Source: CAD feature listing. Evaluate the final solid. Frame: model axes, mm. A direction names the side the tool comes from. Give positions to 0.01 mm unless a question says otherwise; leave off trailing zeros. Write each loop counter-clockwise with the first axis right and the second up, starting at its lowest first coordinate (ties: lowest second). Pieces come first, ordered by that corner, then holes. Notation, with made-up numbers: (53.25, 10.5) -> (84.25, 10.5) arc R28 cw to (84.25, 28.5) -> close; hole circle Ø4 at (63.5, 8.25). An arc over 180 degrees is marked (long way). Answer as a JSON object with one key per item and string values. Group by question number.
Item 1: Section query A-A on y = -3.75. Return the cut outline in (x, z).
Item 2: Ray query, probe 1 along Z at (x, y) = (-10.5, -0.85); probe 2 along X at (y, z) = (-1.85, 207); probe 3 along X at (y, z) = (-2.65, 72). Return the intervals inside material, ascending. Write a range as from..to.
Item 3: First-contact query: pin 1 Ø1.8 at (x, y) = (-14, -1.5) entering from -Z; pin 2 Ø1 at (y, z) = (-3, 9) entering from +X. Flat tips, straight axial feed; report the tip coordinate or a pass-through.
Item 4: Pull-direction query (Z, two-part tool) for faces 4 (the face through (-44, -3, 8)), 5 (the face through (-11, -3, 235)), 6 (the face through (-41, 0, 120)); classes: pulls with the +Z half, pulls with the -Z half, needs draft (parallel to the pull), parting line crosses it, or undercut.
Item 5: Section query B-B on x = -44.5. Return the cut outline in (y, z).
Item 6: Access query for faces 1 (the face through (-39.725, -2.958, 121.903)), 2 (the face through (-41, -3, 4)), 3 (the face through (-46.88, -2.96, 128.19)). Directions: +Z, -Z, +X, -X, +Y, -Y. A direction counts if a zero-diameter tool reaches every point of the face in a straight line with its end or side. Return the directions, or none.
Item 7: Section query C-C on x = -33. Return the cut outline in (y, z).
Item 8: Section query D-D on z = 91.5. Return the cut outline in (x, y), plus the area to 3 significant figures.
from build123d import *

# Parameters (mm, degrees)
F1_DEPTH = 6
F2_DEPTH = 6
F3_DEPTH = 2


with BuildPart() as f1:
    # F0 (on Front) → F1 (new body)
    with BuildSketch(Plane.XZ):
        with BuildLine():
            Line((-17.2, 235), (-4.2, 235))
            Line((-4.2, 235), (-4.2, 241))
            Line((-4.2, 241), (-23.5591068412, 241))
            ThreePointArc((-23.5591068412, 241), (-47.1037067536, 126.5649280043), (-55, 10))
            Line((-55, 10), (-55, 0))
            Line((-55, 0), (-47, 0))
            Line((-47, 0), (-47, 10))
            ThreePointArc((-47, 10), (-39.5176123458, 123.4824215462), (-17.2, 235))
        make_face()
    extrude(amount=F1_DEPTH)

    # F2 (add): a face of the model
    f2_faces = [f1.faces().sort_by_distance(p)[0] for p in [
        (-47, -3, 5),
    ]]
    extrude(f2_faces, amount=F2_DEPTH)

    # F3 (cut): a face of the model
    f3_faces = [f1.faces().sort_by_distance(p)[0] for p in [
        (-44, -3, 10),
    ]]
    extrude(f3_faces, amount=-F3_DEPTH, mode=Mode.SUBTRACT)


solid = f1.part
Worked answers:
{
 "1": {"outline": "(-55, 0) -> (-41, 0) -> (-41, 8) -> (-47, 8) -> (-47, 10) arc R864.31 cw to (-17.2, 235) -> (-4.2, 235) -> (-4.2, 241) -> (-23.56, 241) arc R864.31 ccw to (-55, 10) -> close"},
 "2": {"probe 1": "235..241", "probe 2": "-32.25..-24.25", "probe 3": "-52.77..-44.77"},
 "3": {"pin 1": "z = 235", "pin 2": "x = -47"},
 "4": {"face 4": "undercut", "face 5": "pulls with the -Z half", "face 6": "needs draft"},
 "5": {"outline": "(-6, 0) -> (0, 0) -> (0, 8) -> (-6, 8) -> close; (-6, 75.69) -> (0, 75.69) -> (0, 144.31) -> (-6, 144.31) -> close"},
 "6": {"face 1": "+X, +Y, -Y", "face 2": "-Z, +X, +Y, -Y", "face 3": "+Z, -X, +Y, -Y"},
 "7": {"outline": "(-6, 164.93) -> (0, 164.93) -> (0, 203.77) -> (-6, 203.77) -> close"},
 "8": {"outline": "(-51.15, -6) -> (-43.15, -6) -> (-43.15, 0) -> (-51.15, 0) -> close", "area": "48.0 mm^2"}
}
